Verification items for the finished model (mm, model axes). A direction names the side the tool comes from. Give positions to 0.01 mm unless a question says otherwise; leave off trailing zeros. Answer as a JSON object with one key per item and string values.
```python
from build123d import *

# Parameters (mm, degrees)
SKETCH2_W           = 50
SKETCH2_H           = 150
BOSS_EXTRUDE1_DEPTH = 30
FILLET1_R           = 2
SKETCH3_R           = 13
CUT_EXTRUDE1_DEPTH  = 0.3


with BuildPart() as part:
    # Sketch2 → Boss-Extrude1 (new body)
    with BuildSketch(Plane(origin=(0, 0, 0), x_dir=(1, 0, 0), z_dir=(0, 1, 0))):
        Rectangle(SKETCH2_W, SKETCH2_H)
    extrude(amount=BOSS_EXTRUDE1_DEPTH)

    # Fillet1
    fillet1_edges = [part.edges().sort_by_distance(p)[0] for p in [
        (-25, 30, 0),
        (0, 30, 75),
        (25, 30, 0),
        (0, 0, 75),
        (-25, 0, 0),
        (0, 0, -75),
        (25, 0, 0),
        (25, 15, 75),
        (-25, 15, 75),
        (-25, 15, -75),
        (25, 15, -75),
        (0, 30, -75),
    ]]
    fillet(fillet1_edges, radius=FILLET1_R)

    # Sketch3 → Cut-Extrude1 (cut)
    with BuildSketch(Plane(origin=(0, 0, -75), x_dir=(-1, 0, 0), z_dir=(0, 0, -1))):
        with Locations((0, 15)):
            Circle(SKETCH3_R)
    extrude(amount=-CUT_EXTRUDE1_DEPTH, mode=Mode.SUBTRACT)


solid = part.part
```
(1) Release check for a two-part mould opening along Y. For faces 3 (the flat face through (0, 15, 75)), 4 (the flat face through (0, 0, -1)), 5 (the flat face through (0, 15, -74.7)) record: pulls with the +Y half, pulls with the -Y half, needs draft (parallel to the pull), parting line crosses it, or undercut.
Computed values:
{"face 3": "needs draft", "face 4": "pulls with the -Y half", "face 5": "undercut"}
(2) Material ranges on line 1 along Z through (x, y) = (-4.5, 6.5); line 2 along Y through (x, z) = (0, -74.8); line 3 along X through (y, z) = (15, -74.75), recorded low to high. Write a range as [from, to].
Computed values:
{"line 1": "z = [-74.7, 75]", "line 2": "y = [1.13, 2], [28, 28.87]", "line 3": "x = [-23.97, -13], [13, 23.97]"}
(3) Access from +Z, -Z, +X, -X, +Y, -Y to the whole of each face (thin tool, end or side, straight path). Record for faces 1 (the flat face through (25, 15, 1)), 2 (the cylindrical face through (9.58, 23.79, -74.85)).
Computed values:
{"face 1": "+Z, -Z, +X, +Y, -Y", "face 2": "-Z"}
